Work out the finished part from the listing and answer in its coordinate system (mm). A direction names the side the tool comes from. Coordinates: 2 decimals unless noted, no trailing zeros. Order: outer loops, then holes, each group sorted by start corner. A loop starts at its lowest first (then second) coordinate and runs counter-clockwise, first axis right, second up. Notation, with made-up numbers: (59, -36.75) -> (90, -36.75) arc R8 ccw to (90, -27.75) -> close; hole circle Ø7 at (46, 32.25). An arc over 180 degrees is marked (long way). Write item = value, one per line. Start each with the question number.
Q1. Flat-ended cylindrical pins translate along their axes: pin 1 (1.9 mm diameter, centred on y = 3.5, z = -27.5, fed in from -X); pin 2 (1.9 mm diameter, centred on x = 89, y = 2, fed in from +Z). Find the tip coordinate at first contact, or state that the pin passes through.
Q2. The part is cut by section A-A, the plane z = -36.59. Determine the outline of the cut face in (x, y), plus the area to 3 significant figures.
Q3. The part is cut by section D-D, the plane x = 57.5. Determine the outline of the cut face in (y, z).
Q4. Which of the six approach directions +Z, -Z, +X, -X, +Y, -Y give full straight-line access (tool end or side, diameter ignored) to faces 1 (the flat face through (148, 6.35, -89)), 2 (the flat face through (69, 3, -60))?
Q5. The part is cut by section C-C, the plane z = -146. Determine the outline of the cut face in (x, y), plus the area to 3 significant figures.
Q6. Straight lines are drawn through the part: L1, parallel to Z at x = 170.6, y = 1.75; L2, parallel to X at y = 4.75, z = -77.4; L3, parallel to X at y = 5.5, z = -34. For each, find the intervals that lie inside material, in ascending order. Write a range as from..to.
Q7. For a pull along Z with two mould halves and no side action, classify faces 3 (the cylindrical face through (130.095, 3.131, -104.085)), 4 (the flat face through (192, 3, 0)), 5 (the flat face through (213.048, 3.131, -86.275)) as +Z half, -Z half, draft (parallel to the pull), parting line (faces both ways), or undercut.
Q8. The part is cut by section B-B, the plane y = 4. Count the separate pieces of the cut face and the enclosed holes in it, plus the area to 3 significant figures.
```python
from build123d import *

# Parameters (mm, degrees)
SKETCH1_R           = 5
BOSS_EXTRUDE2_DEPTH = 6.35
SKETCH3_R           = 1.5
CUT_EXTRUDE1_DEPTH  = 6.35
SKETCH4_R           = 2
CUT_EXTRUDE2_DEPTH  = 10
SKETCH6_R           = 2
CUT_EXTRUDE3_DEPTH  = 6.35


with BuildPart() as part:
    # Sketch1 → Boss-Extrude2 (new body)
    with BuildSketch(Plane(origin=(0, 0, 0), x_dir=(1, 0, 0), z_dir=(0, 1, 0))):
        Polygon((180.6, 175), (160.6, 175), (0, 80), (0, 60), (70.5, 60), (140, 60), (140, 0), (194.75, 0), (244.6, 0), align=None)
        with Locations(Location((194.75, 36.59, 0), (0, 0, 270))):
            Circle(SKETCH1_R, mode=Mode.SUBTRACT)
        with BuildLine():
            ThreePointArc((75.5, 81.59), (74.035533906, 78.054466094), (70.5, 76.59))
            ThreePointArc((70.5, 76.59), (66.964466094, 85.125533906), (75.5, 81.59))
        make_face(mode=Mode.SUBTRACT)
        with Locations(Location((129.875, 99.09, 0), (0, 0, 270))):
            Circle(SKETCH1_R, mode=Mode.SUBTRACT)
    extrude(amount=BOSS_EXTRUDE2_DEPTH)

    # Sketch3 → Cut-Extrude1 (cut)
    with BuildSketch(Plane(origin=(0, 6.35, 0), x_dir=(1, 0, 0), z_dir=(0, 1, 0))):
        with Locations(Location((42.27958751, 99.09440108, 0), (0, 0, 270))):
            Circle(SKETCH3_R)
        with Locations(Location((196.359761891, 12, 0), (0, 0, 270))):
            Circle(SKETCH3_R)
        with Locations(Location((228.211428571, 12, 0), (0, 0, 270))):
            Circle(SKETCH3_R)
        with Locations(Location((212.285595231, 55.54720054, 0), (0, 0, 270))):
            Circle(SKETCH3_R)
        with Locations(Location((196.359761891, 99.09440108, 0), (0, 0, 270))):
            Circle(SKETCH3_R)
        with Locations(Location((102.27958751, 99.09440108, 0), (0, 0, 270))):
            Circle(SKETCH3_R)
        with Locations(Location((72.27958751, 99.09440108, 0), (0, 0, 270))):
            Circle(SKETCH3_R)
    extrude(amount=-CUT_EXTRUDE1_DEPTH, mode=Mode.SUBTRACT)

    # Sketch4 → Cut-Extrude2 (cut)
    with BuildSketch(Plane(origin=(0, 6.35, 0), x_dir=(1, 0, 0), z_dir=(0, 1, 0))):
        with BuildLine():
            ThreePointArc((172.6, 160), (172.014213562, 161.414213562), (170.6, 162))
            Line((170.6, 162), (170.6, 160))
            Line((170.6, 160), (170.6, 158))
            ThreePointArc((170.6, 158), (172.014213562, 158.585786438), (172.6, 160))
        make_face()
        with BuildLine():
            Line((170.6, 160), (170.6, 162))
            ThreePointArc((170.6, 162), (168.6, 160), (170.6, 158))
            Line((170.6, 158), (170.6, 160))
        make_face()
        with Locations(Location((170.6, 137.5, 0), (0, 0, 270))):
            Circle(SKETCH4_R)
        with Locations(Location((170.6, 92.5, 0), (0, 0, 270))):
            Circle(SKETCH4_R)
        with Locations(Location((170.6, 47.5, 0), (0, 0, 270))):
            Circle(SKETCH4_R)
        with Locations(Location((170.6, 25, 0), (0, 0, 270))):
            Circle(SKETCH4_R)
    extrude(amount=-CUT_EXTRUDE2_DEPTH, mode=Mode.SUBTRACT)

    # Sketch6 → Cut-Extrude3 (cut)
    with BuildSketch(Plane(origin=(0, 0, 0), x_dir=(-1, 0, 0), z_dir=(0, -1, 0))):
        with Locations(Location((-132, 77.4, 0), (0, 0, 90))):
            Circle(SKETCH6_R)
        with Locations(Location((-108, 77.4, 0), (0, 0, 90))):
            Circle(SKETCH6_R)
        with Locations(Location((-33, 77.4, 0), (0, 0, 90))):
            Circle(SKETCH6_R)
        with Locations(Location((-9, 77.4, 0), (0, 0, 90))):
            Circle(SKETCH6_R)
    extrude(amount=-CUT_EXTRUDE3_DEPTH, mode=Mode.SUBTRACT)


solid = part.part
```
Model answer:
q1.pin_1 = 140
q1.pin_2 = -60
q2.outline = (140, 0) -> (189.75, 0) -> (189.75, 6.35) -> (140, 6.35) -> close; (199.75, 0) -> (231.22, 0) -> (231.22, 6.35) -> (199.75, 6.35) -> close
q2.area = 516 mm2
q3.outline = (0, -114.01) -> (6.35, -114.01) -> (6.35, -60) -> (0, -60) -> close
q4.face_1 = +Z, -Z, +X, -X, +Y
q4.face_2 = +Z, -X, +Y, -Y
q5.outline = (111.57, 0) -> (191.21, 0) -> (191.21, 6.35) -> (111.57, 6.35) -> close
q5.area = 506 mm2
q6.L1 = -175..-162, -158..-139.5, -135.5..-94.5, -90.5..-49.5, -45.5..-27, -23..0
q6.L2 = 0..7, 11..31, 35..67.77, 73.23..106, 110..130, 134..216.29
q6.L3 = 140..190.47, 199.03..232.17
q7.face_3 = undercut
q7.face_4 = +Z half
q7.face_5 = -Z half
q8.separate_pieces = 1
q8.enclosed_holes = 19
q8.area = 20,800 mm2
